Build history of the part. All positions in model axes, mm. Round coordinates to 2 decimals unless told otherwise and drop trailing zeros. Write each loop counter-clockwise with the first axis right and the second up, starting at its lowest first coordinate (ties: lowest second). Pieces come first, ordered by that corner, then holes.
Item 1: Drop flat-ended pins along their axis: pin 1 Ø1 at (x, y) = (-2.5, -69) entering from +Z (3 decimals); pin 2 Ø1.6 at (x, z) = (-2, 40.5) entering from -Y. Give the stop position or say it passes through.
Item 2: Band-saw the part on A-A, the plane x = -1.8. Write the cut outline in (y, z) (1 decimal).
Item 3: Band-saw the part on B-B, the plane z = -97.5. Write the cut outline in (x, y) (3 decimals).
Item 4: Wall check: probe 1 along Y at (x, z) = (-2.35, -97.5). Give the ranges that are in metal, low to high.
```python
from build123d import *

# Parameters (mm, degrees)
SKETCH1_W           = 464.185
SKETCH1_H           = 135.4455
BASE_FLANGE1_DEPTH  = 3.175
SKETCH2_W           = 60.325
SKETCH2_H           = 3.175
BOSS_EXTRUDE2_DEPTH = 3.175


# Sheet-metal steps are written as plain solids
with BuildPart() as part:
    # Sketch1 → Base-Flange1 (new body)
    with BuildSketch(Plane(origin=(0, 0, 0), x_dir=(0, 0, -1), z_dir=(1, 0, 0))):
        Rectangle(SKETCH1_W, SKETCH1_H)
    extrude(amount=-BASE_FLANGE1_DEPTH)

    # Sketch2 → Boss-Extrude2 (add)
    with BuildSketch(Plane(origin=(0, 0, 0), x_dir=(0, 0, -1), z_dir=(1, 0, 0))):
        with Locations((-181.2925, -69.31025)):
            Rectangle(SKETCH2_W, SKETCH2_H)
        with Locations((181.2925, -69.31025)):
            Rectangle(SKETCH2_W, SKETCH2_H)
    extrude(amount=-BOSS_EXTRUDE2_DEPTH)


solid = part.part
```
Results:
1. pin 1: stops at z = 211.455
1. pin 2: stops at y = -67.72
2. outline: (-70.9, -211.5) - (-67.7, -211.5) - (-67.7, -232.1) - (67.7, -232.1) - (67.7, 232.1) - (-67.7, 232.1) - (-67.7, 211.5) - (-70.9, 211.5) - (-70.9, 151.1) - (-67.7, 151.1) - (-67.7, -151.1) - (-70.9, -151.1) - close
3. outline: (-3.175, -67.723) - (0, -67.723) - (0, 67.723) - (-3.175, 67.723) - close
4. probe 1: y = -67.72 to 67.72
